Part model, mm, in its own coordinate system. A direction names the side the tool comes from. Give positions to 0.01 mm unless a question says otherwise; leave off trailing zeros. Order: outer loops, then holes, each group sorted by start corner. A loop starts at its lowest first (then second) coordinate and runs counter-clockwise, first axis right, second up. Notation, with made-up numbers: M 6,76.5 L 43,76.5 A30 ccw 43,99.5 Z; hole C 81.5,76 d7. An arc over 180 degrees is marked long. Write each question's results on one line, items separated by ' | '. Start each with the question number.
from build123d import *

# Parameters (mm, degrees)
ESQUISSE1_W        = 190
ESQUISSE1_H        = 12
BOSS_EXTRU_1_DEPTH = 2.5
CONG_2_R           = 1


with BuildPart() as part:
    # Esquisse1 → Boss.-Extru.1 (new body, symmetric)
    with BuildSketch(Plane(origin=(0, 0, 0), x_dir=(1, 0, 0), z_dir=(0, 1, 0))):
        Rectangle(ESQUISSE1_W, ESQUISSE1_H)
        with BuildLine():
            Line((-88, 2.5), (88, 2.5))
            ThreePointArc((88, 2.5), (90.5, 0), (88, -2.5))
            Line((88, -2.5), (-88, -2.5))
            ThreePointArc((-88, -2.5), (-90.5, 0), (-88, 2.5))
        make_face(mode=Mode.SUBTRACT)
    extrude(amount=BOSS_EXTRU_1_DEPTH, both=True)

    # Congé2
    cong_2_edges = [part.edges().sort_by_distance(p)[0] for p in [
        (95, 0, 6),
        (-95, 0, 6),
        (-95, 0, -6),
        (95, 0, -6),
    ]]
    fillet(cong_2_edges, radius=CONG_2_R)


solid = part.part
(1) Tool access for faces 5 (the flat face through (-1, -2.5, -3)), 6 (the flat face through (-1, 0, -2.5)): list every direction of +Z, -Z, +X, -X, +Y, -Y with a clear straight run to the whole face (end or side of a thin tool).
(2) Saw through at A-A on z = 0. Give the cut face in (x, y), plus the area to 3 significant figures.
(3) Probe L1, parallel to Z at x = -41.5, y = 1.55; L2, parallel to X at y = 0.45, z = 0; L3, parallel to X at y = -0.5, z = 5.25. List the from-to ranges inside material, lowest first.
(4) Saw through at C-C on x = 72. Give the cut face in (y, z).
(5) Saw through at B-B on y = 0.7. Give the cut face in (x, z), plus the area to 3 significant figures.
(6) Pull direction X, two halves, no side cores. Call faces 1 (the cylindrical face through (90.5, 0, -0.1)), 2 (the flat face through (1, 0, 2.5)), 3 (the flat face through (-1, 0, 6)), 4 (the flat face through (95, 0, 0)): +X half, -X half, draft (parallel to the pull), parting line (faces both ways), or undercut.
(7) Drop a flat-ended pin along its axis: P1, Ø2, axis at x = 30.5, z = 0, coming from the +Y side. Give the stop position or say it passes through.
Taken from the geometry:
1) face 5: +Z, -Z, +X, -X, -Y | face 6: +Y, -Y
2) outline: M -95,-2.5 L -90.5,-2.5 L -90.5,2.5 L -95,2.5 Z; M 90.5,-2.5 L 95,-2.5 L 95,2.5 L 90.5,2.5 Z | area: 45.0 mm²
3) L1: z = -6 to -2.5, 2.5 to 6 | L2: x = -95 to -90.5, 90.5 to 95 | L3: x = -94.97 to 94.97
4) outline: M -2.5,-6 L 2.5,-6 L 2.5,-2.5 L -2.5,-2.5 Z; M -2.5,2.5 L 2.5,2.5 L 2.5,6 L -2.5,6 Z
5) outline: M -95,-5 A1 ccw -94,-6 L 94,-6 A1 ccw 95,-5 L 95,5 A1 ccw 94,6 L -94,6 A1 ccw -95,5 Z; hole M -88,-2.5 L 88,-2.5 A2.5 ccw 88,2.5 L -88,2.5 A2.5 ccw Z | area: 1,380 mm²
6) face 1: undercut | face 2: undercut | face 3: draft | face 4: +X half
7) P1: passes through
